from build123d import *

# Parameters (mm, degrees)
F1_DEPTH = 20
F3_DEPTH = 5


with BuildPart() as f1:
    # F0 (on Front) → F1 (new body)
    with BuildSketch(Plane.XZ):
        Polygon((-50, 5), (-50, 0), (50, 0), (50, 5), (5, 5), (-5, 5), align=None)
        Polygon((-5, 73.235), (-5, 5), (5, 5), (5, 73.235), (12.5, 77.565127), (12.5, 85.765), (8.235, 85.765), (8.235, 84.765), (11, 82), (8.235, 79.235), (0, 79.235), (-8.235, 79.235), (-11, 82), (-8.235, 84.765), (-8.235, 85.765), (-12.5, 85.765), (-12.5, 77.565127), align=None)
    extrude(amount=F1_DEPTH)

    # F2 (on face) → F3 (join)
    with BuildSketch(Plane.XZ.offset(20)):
        Polygon((-5, 5), (-50, 5), (-50, 0), (50, 0), (50, 5), (5, 5), align=None)
    extrude(amount=F3_DEPTH)


solid = f1.part
Geometry check sheet. Reference: the model listing, model coordinates, mm. A direction names the side the tool comes from. Give positions to 0.01 mm unless a question says otherwise; leave off trailing zeros. Write each loop counter-clockwise with the first axis right and the second up, starting at its lowest first coordinate (ties: lowest second). Pieces come first, ordered by that corner, then holes. Notation, with made-up numbers: M -26.5,-2.5 L 25.5,-2.5 A19 ccw 25.5,31.5 Z; hole C 24,81 d10. An arc over 180 degrees is marked long. One line per question, with ' | ' between items.
1. Gauge pin test, flat ends, axial feed: pin 1 (2 mm diameter, centred on x = 4, z = 67, fed in from -Y); pin 2 (0.8 mm diameter, centred on y = -11, z = 85, fed in from +X); pin 3 (8 mm diameter, centred on x = 4.5, y = -14, fed in from +Z) (3 decimals); pin 4 (2.5 mm diameter, centred on y = -9, z = 81, fed in from -X). Record the tip position at first contact, or that the pin passes through.
Ans:
pin 1: y = -20 | pin 2: x = 12.5 | pin 3: z = 85.765 | pin 4: x = -12.5
2. Cross-section at D-D (x = 35.5). Enter the section's corners in (y, z).
Ans:
outline: M -25,0 L 0,0 L 0,5 L -25,5 Z
3. Cross-section at B-B (x = 1). Enter the section's corners in (y, z) (3 decimals).
Ans:
outline: M -25,0 L 0,0 L 0,79.235 L -20,79.235 L -20,5 L -25,5 Z
4. Scan lines: line 1 along Z through (x, y) = (0, -19.75) (3 decimals); line 2 along X through (y, z) = (-1, 46); line 3 along Z through (x, y) = (-9.5, -10) (3 decimals). Record each from-to range of solid material in increasing order. Write a range as from..to.
Ans:
line 1: 0..79.235 | line 2: -5..5 | line 3: 0..5, 75.833..80.5, 83.5..85.765
5. Cross-section at A-A (y = -7.75). Enter the section's corners in (x, z) (3 decimals).
Ans:
outline: M -50,0 L 50,0 L 50,5 L 5,5 L 5,73.235 L 12.5,77.565 L 12.5,85.765 L 8.235,85.765 L 8.235,84.765 L 11,82 L 8.235,79.235 L -8.235,79.235 L -11,82 L -8.235,84.765 L -8.235,85.765 L -12.5,85.765 L -12.5,77.565 L -5,73.235 L -5,5 L -50,5 Z
6. Set-up check for faces 1 (the face through (0, -20, 46)), 2 (the face through (0, -10, 79.235)), 3 (the face through (-10, -10, 83)), 4 (the face through (8.7, -9.86, 75.37)), 5 (the face through (-8.8, -9.86, 75.43)): record each of +Z, -Z, +X, -X, +Y, -Y from which the full face is reachable in a straight line by a thin tool's end or side.
Ans:
face 1: +Z, +X, -X, -Y | face 2: +Z, +Y, -Y | face 3: +Y, -Y | face 4: +X, +Y, -Y | face 5: -X, +Y, -Y
7. Mould release check, pull along X, two halves, no side actions. Record for faces 6 (the face through (-50, -12, 3)), 7 (the face through (0, 0, 30)), 8 (the face through (10, -10, 81)): released by +X, released by -X, zero draft, split by the parting line, or undercut.
Ans:
face 6: released by -X | face 7: zero draft | face 8: undercut
8. Cross-section at C-C (z = 64.5). Enter the section's corners in (x, y).
Ans:
outline: M -5,-20 L 5,-20 L 5,0 L -5,0 Z
